Geometry check sheet. Reference: the model listing, model coordinates, mm. A direction names the side the tool comes from. Round coordinates to 2 decimals unless told otherwise and drop trailing zeros. Order: outer loops, then holes, each group sorted by start corner. A loop starts at its lowest first (then second) coordinate and runs counter-clockwise, first axis right, second up.
Autodesk Inventor part; units mm, degrees
ref_plane "YZ Plane" through (0, 0, 0) normal (1, 0, 0) x (0, 1, 0)
ref_plane "XZ Plane" through (0, 0, 0) normal (0, 1, 0) x (-1, 0, 0)
ref_plane "XY Plane" through (0, 0, 0) normal (0, 0, 1) x (1, 0, 0)
sketch "Skizze_1" plane through (0, 0, 0) normal (0, 0, 1) x (1, 0, 0)
  arc A0 (-4.15, 0.2) -> (-3.95, 0) centre (-3.95, 0.2) ccw
  line L0 (-3.95, 0) -> (4.15, 0)
  arc A1 (4.15, 0) -> (4.35, 0.2) centre (4.15, 0.2) ccw
  line L1 (4.35, 0.2) -> (4.35, 10.1)
  arc A2 (4.35, 10.1) -> (4.15, 10.3) centre (4.15, 10.1) ccw
  line L2 (4.15, 10.3) -> (-3.95, 10.3)
  arc A3 (-3.95, 10.3) -> (-4.15, 10.1) centre (-3.95, 10.1) ccw
  line L3 (-4.15, 10.1) -> (-4.15, 0.2)
extrude "Extrusion1" add sketch "Skizze_1" along normal blind 9.4
sketch "Skizze_2" plane through (0, 0, 0.95) normal (0, 0, 1) x (1, 0, 0)
  line L0 (-2.35, 10.3) -> (-2.35, 2.6)
  line L1 (-2.35, 2.6) -> (2.35, 2.6)
  line L2 (2.35, 2.6) -> (2.35, 10.3)
  line L3 (2.35, 10.3) -> (-2.35, 10.3)
extrude "Extrusion2" cut sketch "Skizze_2" along normal blind 7.5
sketch "Skizze_3" plane through (0, 10.3, 0) normal (0, 1, 0) x (1, 0, 0)
  line L0 (-0.9, -0.95) -> (0.9, -0.95)
  line L1 (0.9, -0.95) -> (0.9, -0.65)
  line L2 (0.9, -0.65) -> (-0.9, -0.65)
  line L3 (-0.9, -0.65) -> (-0.9, -0.95)
extrude "Extrusion3" cut sketch "Skizze_3" against normal blind 7.7
sketch "Skizze_4" plane through (0, 10.3, 0) normal (0, 1, 0) x (1, 0, 0)
  line L0 (-0.9, -8.45) -> (-0.9, -8.75)
  line L1 (-0.9, -8.75) -> (0.9, -8.75)
  line L2 (0.9, -8.75) -> (0.9, -8.45)
  line L3 (0.9, -8.45) -> (-0.9, -8.45)
extrude "Extrusion4" cut sketch "Skizze_4" against normal blind 7.7
sketch "Skizze_5" plane through (0, 10.3, 0) normal (0, 1, 0) x (1, 0, 0)
  line L0 (2.35, -0.95) -> (2.35, -2.9)
  line L1 (2.35, -2.9) -> (3.95, -2.9)
  line L2 (3.95, -2.9) -> (3.95, -0.95)
  line L3 (3.95, -0.95) -> (2.35, -0.95)
extrude "Extrusion5" cut sketch "Skizze_5" against normal blind 6
sketch "Skizze_6" plane through (0, 10.3, 0) normal (0, 1, 0) x (1, 0, 0)
  line L0 (2.35, -6.7) -> (3.95, -6.7)
  line L1 (3.95, -6.7) -> (3.95, -4.75)
  line L2 (3.95, -4.75) -> (2.35, -4.75)
  line L3 (2.35, -4.75) -> (2.35, -6.7)
extrude "Extrusion6" cut sketch "Skizze_6" against normal blind 6
sketch "Skizze_7" plane through (0, 0, 0) normal (0, 1, 0) x (-1, 0, 0)
  line L0 (1.4, 1.7) -> (1.4, 4.5)
  line L1 (1.4, 4.5) -> (-1.4, 4.5)
  line L2 (-1.4, 4.5) -> (-1.4, 1.7)
  line L3 (-1.4, 1.7) -> (1.4, 1.7)
extrude "Extrusion7" add sketch "Skizze_7" along normal blind 3.6
pattern_linear "Rectangular Pattern1" count 2 spacing 3.5 along (0, 0, 1) of "Extrusion7"
sketch "Skizze_9" plane through (0, 0, 0) normal (0, 1, 0) x (-1, 0, 0)
  line L0 (0.5, 2.6) -> (0.5, 3.6)
  line L1 (0.5, 3.6) -> (-0.5, 3.6)
  line L2 (-0.5, 3.6) -> (-0.5, 2.6)
  line L3 (-0.5, 2.6) -> (0.5, 2.6)
extrude "Extrusion8" add sketch "Skizze_9" along normal blind 9.3
pattern_linear "Rectangular Pattern2" count 2 spacing 3.5 along (0, 0, 1) of "Extrusion8"
sketch "Skizze_11" plane through (0, 0, 0) normal (0, 1, 0) x (-1, 0, 0)
  line L0 (0.5, 2.6) -> (0.5, 3.6)
  line L1 (0.5, 3.6) -> (-0.5, 3.6)
  line L2 (-0.5, 3.6) -> (-0.5, 2.6)
  line L3 (-0.5, 2.6) -> (0.5, 2.6)
extrude "Extrusion9" add sketch "Skizze_11" against normal blind 4.5
pattern_linear "Rectangular Pattern3" count 2 spacing 3.5 along (0, 0, 1) of "Extrusion9"
sketch "Skizze_13" plane through (0, 0, 0) normal (0, 1, 0) x (-1, 0, 0)
  line L0 (2.75, 0) -> (2.75, 0.4)
  line L1 (2.75, 0.4) -> (0.9, 0.4)
  line L2 (0.9, 0.4) -> (0.9, 0.65)
  line L3 (0.9, 0.65) -> (-0.9, 0.65)
  line L4 (-0.9, 0.65) -> (-0.9, 0.4)
  line L5 (-0.9, 0.4) -> (-2.75, 0.4)
  line L6 (-2.75, 0.4) -> (-2.75, 0)
  line L7 (-2.75, 0) -> (2.75, 0)
extrude "Extrusion10" cut sketch "Skizze_13" along normal blind 8.3
sketch "Skizze_14" plane through (0, 0, 0) normal (0, 1, 0) x (-1, 0, 0)
  line L0 (2.75, 9.4) -> (-2.75, 9.4)
  line L1 (-2.75, 9.4) -> (-2.75, 9)
  line L2 (-2.75, 9) -> (-0.9, 9)
  line L3 (-0.9, 9) -> (-0.9, 8.75)
  line L4 (-0.9, 8.75) -> (0.9, 8.75)
  line L5 (0.9, 8.75) -> (0.9, 9)
  line L6 (0.9, 9) -> (2.75, 9)
  line L7 (2.75, 9) -> (2.75, 9.4)
extrude "Extrusion11" cut sketch "Skizze_14" along normal blind 8.3
sketch "Skizze_15" plane through (0, 0, 0) normal (0, 1, 0) x (-1, 0, 0)
  line L0 (4.15, 1.8) -> (4.15, 4.4)
  line L1 (4.15, 4.4) -> (2.95, 4.4)
  line L2 (2.95, 4.4) -> (2.95, 1.8)
  line L3 (2.95, 1.8) -> (4.15, 1.8)
extrude "Extrusion12" cut sketch "Skizze_15" along normal blind 9.15
pattern_linear "Rectangular Pattern4" count 2 spacing 3.5 along (0, 0, 1) of "Extrusion12"
sketch "Skizze_17" plane through (0, 0, 0) normal (0, 1, 0) x (-1, 0, 0)
  line L0 (-3.55, 2.55) -> (-3.55, 3.65)
  line L1 (-3.55, 3.65) -> (-4.05, 3.65)
  line L2 (-4.05, 3.65) -> (-4.05, 4.4)
  line L3 (-4.05, 4.4) -> (-4.35, 4.4)
  line L4 (-4.35, 4.4) -> (-4.35, 1.8)
  line L5 (-4.35, 1.8) -> (-4.05, 1.8)
  line L6 (-4.05, 1.8) -> (-4.05, 2.55)
  line L7 (-4.05, 2.55) -> (-3.55, 2.55)
extrude "Extrusion13" cut sketch "Skizze_17" along normal blind 3.9
sketch "Skizze_18" plane through (0, 0, 0) normal (0, 1, 0) x (-1, 0, 0)
  line L0 (-3.55, 6.05) -> (-3.55, 7.15)
  line L1 (-3.55, 7.15) -> (-4.05, 7.15)
  line L2 (-4.05, 7.15) -> (-4.05, 7.9)
  line L3 (-4.05, 7.9) -> (-4.35, 7.9)
  line L4 (-4.35, 7.9) -> (-4.35, 5.3)
  line L5 (-4.35, 5.3) -> (-4.05, 5.3)
  line L6 (-4.05, 5.3) -> (-4.05, 6.05)
  line L7 (-4.05, 6.05) -> (-3.55, 6.05)
extrude "Extrusion14" cut sketch "Skizze_18" along normal blind 3.9
sketch "Sketch15" plane through (-0.5, 9.3, 6.1) normal (0, 1, 0) x (1, 0, 0)
  line L0 (0, 0) -> (1, 0)
  line L1 (0, -1) -> (0, 0)
  line L2 (1, -1) -> (0, -1)
  line L3 (1, 0) -> (1, -1)
  line L4 (0, -1) -> (1, 0) construction
  point P0 (0.5, 6.1)
  point P1 (0.5, -0.5)
sketch "Sketch16" plane through (-0.5, 9.3, 6.1) normal (0, 1, 0) x (1, 0, 0)
  line L0 (0, 3.5) -> (1, 3.5) construction
  line L1 (0, 2.5) -> (0, 3.5) construction
  line L2 (1, 2.5) -> (0, 2.5) construction
  line L3 (1, 3.5) -> (1, 2.5) construction
  line L4 (0, 0) -> (1, 0) construction
  line L5 (0, -1) -> (0, 0) construction
  line L6 (1, -1) -> (0, -1) construction
  line L7 (1, 0) -> (1, -1) construction
  line L8 (1, -1) -> (0, 0) construction
  line L9 (1, 2.5) -> (0, 3.5) construction
  circle A0 centre (0.5, 3) radius 0.25
  circle A1 centre (0.5, -0.5) radius 0.25
  point P0 (0.5, 6.1)
  dimension "d52" = 0.5
extrude "Extrusion15" cut sketch "Sketch16" against normal through all
properties part number "Wago Power In"
(1) Material ranges on line 1 (Z direction, x = 0, y = 2.5); line 2 (Z direction, x = 0, y = 4.5); line 3 (X direction, y = 4.75, z = 6.6), recorded low to high.
Returned:
line 1: z = 0.65 to 2.85, 3.35 to 6.35, 6.85 to 8.75
line 2: z = 2.6 to 2.85, 3.35 to 3.6, 6.1 to 6.35, 6.85 to 7.1
line 3: x = -2.95 to -2.35, -0.5 to -0.25, 0.25 to 0.5, 3.95 to 4.35
(2) Sectioned sample at C-C, the plane x = 1.75. Record the cut outline in (y, z).
Returned:
outline: (0, 0.4) - (8.3, 0.4) - (8.3, 0) - (10.3, 0) - (10.3, 0.95) - (2.6, 0.95) - (2.6, 8.45) - (10.3, 8.45) - (10.3, 9.4) - (8.3, 9.4) - (8.3, 9) - (0, 9) - close
(3) Sectioned sample at D-D, the plane z = 5.75. Record the cut outline in (x, y), and give its area (3 significant figures).
Returned:
outline: (-4.15, 9.15) - (-2.95, 9.15) - (-2.95, 0) - (4.05, 0) - (4.05, 3.9) - (4.35, 3.9) - (4.35, 10.1) arc R0.2 ccw to (4.15, 10.3) - (3.95, 10.3) - (3.95, 4.3) - (2.35, 4.3) - (2.35, 2.6) - (1.4, 2.6) - (1.4, 3.6) - (-1.4, 3.6) - (-1.4, 2.6) - (-2.35, 2.6) - (-2.35, 10.3) - (-3.95, 10.3) arc R0.2 ccw to (-4.15, 10.1) - close
area: 32.4 mm2
(4) Set-up check for faces 1 (the flat face through (0, -2, 3.6)), 2 (the flat face through (0, -2, 7.1)), 3 (the flat face through (0.5, -2, 3)), 4 (the flat face through (2.35, 5.5, 4.6)): record each of +Z, -Z, +X, -X, +Y, -Y from which the full face is reachable in a straight line by a thin tool's end or side.
Returned:
face 1: +X, -X, -Y
face 2: +Z, +X, -X, -Y
face 3: +Z, -Z, +X, -Y
face 4: +Y
(5) Draft check along Z on faces 5 (the flat face through (2, 4, 9)), 6 (the flat face through (0, -2, 6.1)), 7 (the flat face through (-2, 7, 8.45)), 8 (the flat face through (-0.5, -2, 3)). Enter one of: released by +Z, released by -Z, zero draft, split by the parting line, or undercut.
Returned:
face 5: released by +Z
face 6: undercut
face 7: undercut
face 8: zero draft
(6) Depth check by flat-ended pin: P1, Ø1.1, axis at y = -3, z = 6.5, coming from the +X side; P2, Ø1.4, axis at x = 0.5, z = 2.5, coming from the +Y side; P3, Ø0.8, axis at y = 7, z = 7, coming from the -X side. Enter the tip coordinate at first touch or a pass-through.
Returned:
P1: stops at x = 0.5
P2: stops at y = 9.3
P3: stops at x = -2.95
(7) Sectioned sample at A-A, the plane y = -3.5. Record the cut outline in (x, z).
Returned:
outline: (-0.5, 2.6) - (0.5, 2.6) - (0.5, 3.6) - (-0.5, 3.6) - close; (-0.5, 6.1) - (0.5, 6.1) - (0.5, 7.1) - (-0.5, 7.1) - close; hole circle Ø0.5 at (0, 3.1); hole circle Ø0.5 at (0, 6.6)
